Build history of the part. All positions in model axes, mm. Coordinates: 2 decimals unless noted, no trailing zeros. Order: outer loops, then holes, each group sorted by start corner. A loop starts at its lowest first (then second) coordinate and runs counter-clockwise, first axis right, second up. Notation, with made-up numbers: (46, -18) - (91, -18) arc R17 cw to (91, -11) - close; hole circle Ø6 at (50, 66). An arc over 180 degrees is marked (long way). Write each question's results on one line, items separated by ' | '.
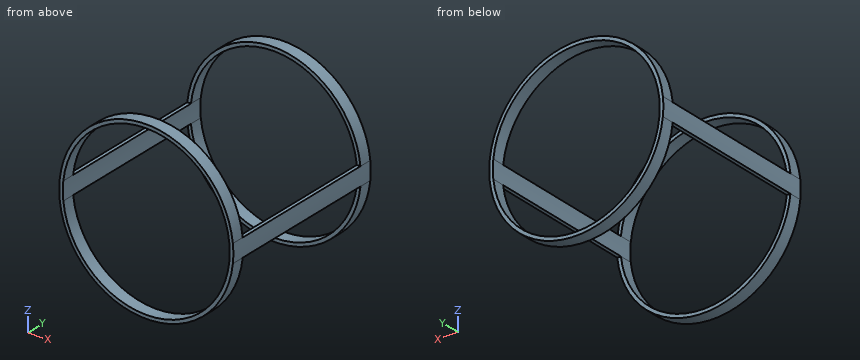
from build123d import *

# Parameters (mm, degrees)
BOSS_EXTRUDE1_DEPTH   = 97.5
BOSS_EXTRUDE1_2_DEPTH = 97.5
SKETCH2_R             = 48.25
SKETCH2_R_2           = 46.25
BOSS_EXTRUDE2_DEPTH   = 7
BOSS_EXTRUDE3_START   = -7
SKETCH3_R             = 48.25
SKETCH3_R_2           = 46.25
BOSS_EXTRUDE3_DEPTH   = 7


with BuildPart() as part:
    # Sketch1 → Boss-Extrude1 (new body)
    with BuildSketch(Plane(origin=(0, 0, 0), x_dir=(1, 0, 0), z_dir=(0, 1, 0))):
        with BuildLine():
            Line((-47.990233381, 5), (-45.978935394, 5))
            ThreePointArc((-45.978935394, 5), (-46.25, 0), (-45.978935394, -5))
            Line((-45.978935394, -5), (-47.990233381, -5))
            ThreePointArc((-47.990233381, -5), (-48.25, 0), (-47.990233381, 5))
        make_face()
    extrude(amount=BOSS_EXTRUDE1_DEPTH)



with BuildPart() as body_2:
    # Sketch1 → Boss-Extrude1 2 (new body)
    with BuildSketch(Plane(origin=(0, 0, 0), x_dir=(1, 0, 0), z_dir=(0, 1, 0))):
        with BuildLine():
            Line((47.990233381, -5), (45.978935394, -5))
            ThreePointArc((45.978935394, -5), (46.25, 0), (45.978935394, 5))
            Line((45.978935394, 5), (47.990233381, 5))
            ThreePointArc((47.990233381, 5), (48.25, 0), (47.990233381, -5))
        make_face()
    extrude(amount=BOSS_EXTRUDE1_2_DEPTH)


with BuildPart() as part_1:
    add(part.part)

    add(body_2.part)  # Boss-Extrude2 merges body 2
    # Sketch2 → Boss-Extrude2 (add)
    with BuildSketch(Plane(origin=(0, 0, 0), x_dir=(1, 0, 0), z_dir=(0, 1, 0))):
        with Locations(Location((0, 0, 0), (0, 0, 5.94806464))):
            Circle(SKETCH2_R)
        with Locations(Location((0, 0, 0), (0, 0, 173.793732249))):
            Circle(SKETCH2_R_2, mode=Mode.SUBTRACT)
    extrude(amount=BOSS_EXTRUDE2_DEPTH)

    # Sketch3 → Boss-Extrude3 (add)
    with BuildSketch(Plane(origin=(0, 97.5, 0), x_dir=(1, 0, 0), z_dir=(0, 1, 0)).offset(BOSS_EXTRUDE3_START)):
        with Locations(Location((0, 0, 0), (0, 0, 270))):
            Circle(SKETCH3_R)
        with Locations(Location((0, 0, 0), (0, 0, 270))):
            Circle(SKETCH3_R_2, mode=Mode.SUBTRACT)
    extrude(amount=BOSS_EXTRUDE3_DEPTH)


solid = part_1.part
1. Band-saw the part on A-A on x = 5. Give the cut face in (y, z).
Solved:
outline: (0, -47.99) - (7, -47.99) - (7, -45.98) - (0, -45.98) - close; (0, 45.98) - (7, 45.98) - (7, 47.99) - (0, 47.99) - close; (90.5, -47.99) - (97.5, -47.99) - (97.5, -45.98) - (90.5, -45.98) - close; (90.5, 45.98) - (97.5, 45.98) - (97.5, 47.99) - (90.5, 47.99) - close
2. Band-saw the part on C-C on z = 21.5. Give the cut face in (x, y), then the cut area to 3 significant figures.
Solved:
outline: (-43.2, 0) - (-40.95, 0) - (-40.95, 7) - (-43.2, 7) - close; (-43.2, 90.5) - (-40.95, 90.5) - (-40.95, 97.5) - (-43.2, 97.5) - close; (40.95, 0) - (43.2, 0) - (43.2, 7) - (40.95, 7) - close; (40.95, 90.5) - (43.2, 90.5) - (43.2, 97.5) - (40.95, 97.5) - close | area: 62.9 mm2
3. Band-saw the part on D-D on z = 2.5. Give the cut face in (x, y).
Solved:
outline: (-48.19, 0) - (-46.18, 0) - (-46.18, 97.5) - (-48.19, 97.5) - close; (46.18, 0) - (48.19, 0) - (48.19, 97.5) - (46.18, 97.5) - close
4. Band-saw the part on B-B on y = 54.5. Give the cut face in (x, z).
Solved:
outline: (-47.99, -5) - (-45.98, -5) arc R46.25 cw to (-45.98, 5) - (-47.99, 5) arc R48.25 ccw to start; (45.98, -5) - (47.99, -5) arc R48.25 ccw to (47.99, 5) - (45.98, 5) arc R46.25 cw to start
5. Drop flat-ended pins along their axis: pin 1 Ø1 at (x, y) = (47, 39) entering from +Z; pin 2 Ø0.6 at (x, y) = (47.5, 37) entering from -Z; pin 3 Ø5 at (y, z) = (40.5, -7) entering from +X. Give the stop position or say it passes through.
Solved:
pin 1: stops at z = 5 | pin 2: stops at z = -5 | pin 3: stops at x = 48.04
6. Probe line 1 (Y direction, x = -43, z = 19); line 2 (X direction, y = 5, z = 28); line 3 (X direction, y = 37.5, z = 4). List the from-to ranges inside material, lowest first.
Solved:
line 1: y = 0 to 7, 90.5 to 97.5 | line 2: x = -39.29 to -36.81, 36.81 to 39.29 | line 3: x = -48.08 to -46.08, 46.08 to 48.08
